Study the drawing (mm; zero at the part's minimum x, y, z) and answer. Coordinates: 2 decimals unless noted, no trailing zeros. Loops run counter-clockwise (first coordinate to the right, second up) from the corner with the lowest first, then second, coordinate; pieces in that order, holes last.
Q1. Straight lines are drawn through the part: line 1 (Z direction, x = 0.75, y = 25) (1 decimal); line 2 (Z direction, x = 1, y = 37.5) (1 decimal); line 3 (Y direction, x = 3.25, z = 4) (1 decimal). For each, find the intervals that lie inside material, in ascending order.
Q2. The mould has two halves that part along Y. Classify the marked faces 1, 2 and 3: pulls with the +Y half, pulls with the -Y half, needs draft (parallel to the pull), parting line crosses it, or undercut.
Q3. Section B-B (x = 3) is taken. Give the vertices of the cut face in (y, z) (1 decimal).
Q4. Section C-C (y = 11) is taken. Give the vertices of the cut face in (x, z), then the cut area to 3 significant figures.
Q5. Flat-ended cylindrical pins translate along their axes: P1, Ø16.5, axis at y = 24.892, z = 24.892, coming from the +X side; P2, Ø2, axis at x = 4, z = 35.5, coming from the +Y side (1 decimal); P3, Ø1.5, axis at x = 1, y = 28.5, coming from the -Z side (1 decimal); P4, Ø3, axis at x = 3, y = 14, coming from the -Z side. Find the tip coordinate at first contact, or state that the pin passes through.
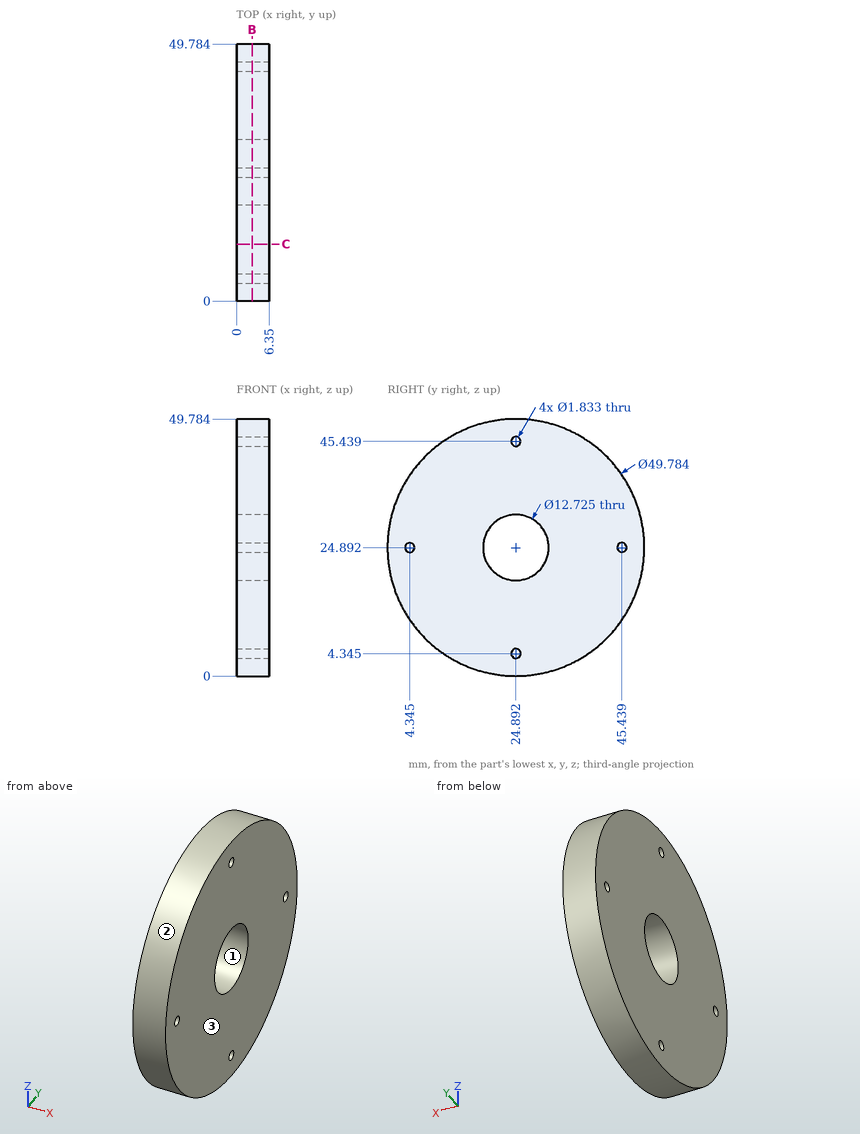
Numbers:
1. line 1: z = 0 to 3.4, 5.3 to 18.5, 31.3 to 44.5, 46.3 to 49.8
1. line 2: z = 3.4 to 46.4
1. line 3: y = 11.4 to 24, 25.7 to 38.4
2. face 1: undercut
2. face 2: parting line crosses it
2. face 3: needs draft
3. outline: circle Ø49.8 at (24.9, 24.9); hole circle Ø1.8 at (4.3, 24.9); hole circle Ø12.7 at (24.9, 24.9); hole circle Ø1.8 at (24.9, 4.3); hole circle Ø1.8 at (24.9, 45.4); hole circle Ø1.8 at (45.4, 24.9)
4. outline: (0, 4.24) - (6.35, 4.24) - (6.35, 45.55) - (0, 45.55) - close
4. area: 262 mm2
5. P1: stops at x = 6.35
5. P2: stops at y = 47.9
5. P3: stops at z = 0.2
5. P4: stops at z = 1.84
